The listing builds one solid part. Answer for the finished solid, in the listing's coordinates (mm). Face numbers are marked on the shaded views. A direction names the side the tool comes from. Give positions to 0.01 mm unless a question says otherwise; leave off trailing zeros. Write each loop counter-clockwise with the first axis right and the second up, starting at its lowest first coordinate (ties: lowest second). Pieces come first, ordered by that corner, then holes. Notation, with made-up numbers: (28, 50) - (48, 50) arc R21 cw to (48, 69) - close; hole circle Ø7 at (15, -15.5). An arc over 180 degrees is marked (long way). Use a Markdown table: item, result. Add a question column.
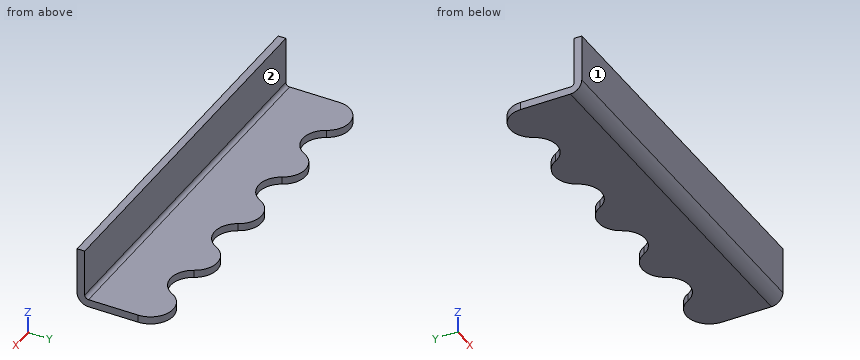
from build123d import *

# Parameters (mm, degrees)
SM_BASE_FLANGE_1_DEPTH           = 1.5
SM_EDGE_FLANGE_1_STRIP_W         = 7.48
SM_EDGE_FLANGE_1_STRIP_H         = 1.5
SM_EDGE_FLANGE_1_STRIP_CUT_DEPTH = 73
SM_EDGE_FLANGE_1_DEPTH           = 73


# Sheet-metal steps are written as plain solids
with BuildPart() as part:
    # Sketch 1 → Базовая кромка1 (new body)
    with BuildSketch(Plane.XY):
        with BuildLine():
            Line((-36.5, 0), (36.5, 0))
            Line((36.5, 0), (36.5, 10.5))
            ThreePointArc((36.5, 10.5), (33.060660172, 14.873213921), (28, 12.561552813))
            ThreePointArc((28, 12.561552813), (24, 10.123105626), (20, 12.561552813))
            ThreePointArc((20, 12.561552813), (16, 15), (12, 12.561552813))
            ThreePointArc((12, 12.561552813), (8, 10.123105626), (4, 12.561552813))
            ThreePointArc((4, 12.561552813), (0, 15), (-4, 12.561552813))
            ThreePointArc((-4, 12.561552813), (-8, 10.123105626), (-12, 12.561552813))
            ThreePointArc((-12, 12.561552813), (-16, 15), (-20, 12.561552813))
            ThreePointArc((-20, 12.561552813), (-24, 10.123105626), (-28, 12.561552813))
            ThreePointArc((-28, 12.561552813), (-33.060660172, 14.873213921), (-36.5, 10.5))
            Line((-36.5, 10.5), (-36.5, 0))
        make_face()
    extrude(amount=-SM_BASE_FLANGE_1_DEPTH)

    # Ребро-кромка1 strip (across the edge) → Ребро-кромка1 strip cut (cut)
    with BuildSketch(Plane.YZ.offset(-36.5)):
        with Locations((-3, -0.75)):
            Rectangle(SM_EDGE_FLANGE_1_STRIP_W, SM_EDGE_FLANGE_1_STRIP_H)
    extrude(amount=SM_EDGE_FLANGE_1_STRIP_CUT_DEPTH, mode=Mode.SUBTRACT)

    # Ребро-кромка1 section (across the edge) → Ребро-кромка1 (add)
    with BuildSketch(Plane.YZ.offset(-36.5)):
        with BuildLine():
            Line((-1.5, 0.74), (-1.5, 10))
            Line((-1.5, 10), (0, 10))
            Line((0, 10), (0, 0.74))
            ThreePointArc((0, 0.74), (0.216740982, 0.216740982), (0.74, 0))
            Line((0.74, 0), (0.74, -1.5))
            ThreePointArc((0.74, -1.5), (-0.84391919, -0.84391919), (-1.5, 0.74))
        make_face()
    extrude(amount=SM_EDGE_FLANGE_1_DEPTH)


solid = part.part
1. Given P1, Ø6, axis at x = 18, y = 4, coming from the +Z side; P2, Ø3, axis at x = -12.5, z = 0, coming from the +Y side, each flat-ended and moving along its own axis, determine where each tip first touches the part or whether it passes through.
2. The part is cut by section D-D (x = -22.5). Give the vertices of the cut face in (y, z), and give its area (3 significant figures).
3. The part is cut by section B-B (x = -31). Give the vertices of the cut face in (y, z), and give its area (3 significant figures).
4. Which of the six approach directions +Z, -Z, +X, -X, +Y, -Y give full straight-line access (tool end or side, diameter ignored) to the marked faces 1 and 2?
5. Consider L1, parallel to Y at x = -31.5, z = 2.5; L2, parallel to Y at x = 27.5, z = -0.75. Determine where each line is inside the solid, lowest interval first. Write a range as [from, to].
6. The part is cut by section C-C (z = 3.5). Give the vertices of the cut face in (x, y), and give its area (4 significant figures).
7. The part is cut by section A-A (y = 11.25). Give the vertices of the cut face in (x, z), and give its area (3 significant figures).
Check values:
| question | item | result |
|---|---|---|
| 1 | P1 | stops at z = 0 |
| 1 | P2 | stops at y = 14.53 |
| 2 | outline | (-1.5, 0.74) arc R2.24 ccw to (0.74, -1.5) - (10.38, -1.5) - (10.38, 0) - (0.74, 0) arc R0.74 cw to (0, 0.74) - (0, 10) - (-1.5, 10) - close |
| 2 | area | 31.9 mm2 |
| 3 | outline | (-1.5, 0.74) arc R2.24 ccw to (0.74, -1.5) - (14.89, -1.5) - (14.89, 0) - (0.74, 0) arc R0.74 cw to (0, 0.74) - (0, 10) - (-1.5, 10) - close |
| 3 | area | 38.6 mm2 |
| 4 | face 1 | +Z, -Z, +X, -X, -Y |
| 4 | face 2 | +Z, +X, -X, +Y |
| 5 | L1 | y = [-1.5, 0] |
| 5 | L2 | y = [-0.93, 11.79] |
| 6 | outline | (-36.5, -1.5) - (36.5, -1.5) - (36.5, 0) - (-36.5, 0) - close |
| 6 | area | 109.5 mm2 |
| 7 | outline | (-36.44, -1.5) - (-26.98, -1.5) - (-26.98, 0) - (-36.44, 0) - close; (-21.02, -1.5) - (-10.98, -1.5) - (-10.98, 0) - (-21.02, 0) - close; (-5.02, -1.5) - (5.02, -1.5) - (5.02, 0) - (-5.02, 0) - close; (10.98, -1.5) - (21.02, -1.5) - (21.02, 0) - (10.98, 0) - close; (26.98, -1.5) - (36.44, -1.5) - (36.44, 0) - (26.98, 0) - close |
| 7 | area | 73.6 mm2 |
